Build history of the part. All positions in model axes, mm. Give positions to 0.01 mm unless a question says otherwise; leave off trailing zeros. Order: outer loops, then holes, each group sorted by start corner. A loop starts at its lowest first (then second) coordinate and runs counter-clockwise, first axis right, second up. Notation, with made-up numbers: (-24, 54) -> (21, 54) arc R19 cw to (21, 79) -> close; hole circle Ø1 at (25, -36). An arc over 180 degrees is marked (long way). Use a Markdown table: item, result. Add a question column.
```python
from build123d import *

# Parameters (mm, degrees)
SALIENTE_EXTRUIR1_DEPTH = 3
CROQUIS2_W              = 16.03671643
CROQUIS2_H              = 6
CORTAR_EXTRUIR1_DEPTH   = 10


with BuildPart() as part:
    # Croquis1 → Saliente-Extruir1 (new body)
    with BuildSketch(Plane(origin=(0, 0, 0), x_dir=(1, 0, 0), z_dir=(0, 1, 0))):
        Polygon((480, 280), (480, 283.1), (460, 283.1), (460, 280), (440, 280), (440, 283.1), (420, 283.1), (420, 280), (400, 280), (400, 283.1), (380, 283.1), (380, 280), (360, 280), (360, 283.1), (340, 283.1), (340, 280), (320, 280), (320, 283.1), (300, 283.1), (300, 280), (280, 280), (280, 283.1), (260, 283.1), (260, 280), (240, 280), (240, 283.1), (220, 283.1), (220, 280), (200, 280), (200, 283.1), (180, 283.1), (180, 280), (160, 280), (160, 283.1), (140, 283.1), (140, 280), (120, 280), (120, 283.1), (100, 283.1), (100, 280), (80, 280), (80, 283.1), (60, 283.1), (60, 280), (40, 280), (40, 283.1), (20, 283.1), (20, 280), (0, 280), (0, 260), (-3.1, 260), (-3.1, 240), (0, 240), (0, 220), (-3.1, 220), (-3.1, 200), (0, 200), (0, 180), (-3.1, 180), (-3.1, 160), (0, 160), (0, 140), (-3.1, 140), (-3.1, 120), (0, 120), (0, 100), (-3.1, 100), (-3.1, 80), (0, 80), (0, 60), (-3.1, 60), (-3.1, 40), (0, 40), (0, 20), (-3.1, 20), (-3.1, 0), (0, 0), (480, 0), (480, 20), (483.1, 20), (483.1, 40), (480, 40), (480, 60), (483.1, 60), (483.1, 80), (480, 80), (480, 100), (483.1, 100), (483.1, 120), (480, 120), (480, 140), (483.1, 140), (483.1, 160), (480, 160), (480, 180), (483.1, 180), (483.1, 200), (480, 200), (480, 220), (483.1, 220), (483.1, 240), (480, 240), (480, 260), (483.1, 260), (483.1, 280), align=None)
    extrude(amount=SALIENTE_EXTRUIR1_DEPTH)

    # Croquis2 → Cortar-Extruir1 (cut)
    with BuildSketch(Plane(origin=(0, 3, 0), x_dir=(1, 0, 0), z_dir=(0, 1, 0))):
        with Locations((270.581641785, 3)):
            Rectangle(CROQUIS2_W, CROQUIS2_H)
    extrude(amount=-CORTAR_EXTRUIR1_DEPTH, mode=Mode.SUBTRACT)


solid = part.part
```
(1) Band-saw the part on A-A on x = 271. Give the cut face in (y, z).
(2) Wall check: probe 1 along Z at (x, y) = (452.5, 2); probe 2 along X at (y, z) = (2.55, -145.5); probe 3 along X at (y, z) = (0.5, -206.5). Give the ranges that are in metal, low to high.
(3) Pin check, flat tips, straight feed: pin 1 Ø0.9 at (y, z) = (1.5, -281) entering from -X; pin 2 Ø1.5 at (y, z) = (1, -282) entering from +X; pin 3 Ø1.5 at (x, y) = (270, 2) entering from +Z. Stop position of each tip, or through.
Response:
| question | item | result |
|---|---|---|
| 1 | outline | (0, -283.1) -> (3, -283.1) -> (3, -6) -> (0, -6) -> close |
| 2 | probe 1 | z = -280 to 0 |
| 2 | probe 2 | x = 0 to 483.1 |
| 2 | probe 3 | x = -3.1 to 480 |
| 3 | pin 1 | stops at x = 20 |
| 3 | pin 2 | stops at x = 480 |
| 3 | pin 3 | stops at z = -6 |
